Job drawing, mm, ordinate dimensions from the low corner. One solid piece. A direction names the side the tool comes from. Coordinates: 2 decimals unless noted, no trailing zeros. Loops run counter-clockwise (first coordinate to the right, second up) from the corner with the lowest first, then second, coordinate; pieces in that order, holes last. Notation, with made-up numbers: (31, 12) -> (37, 12) arc R32 ccw to (37, 42) -> close; hole circle Ø7 at (68, -21.5). An arc over 180 degrees is marked (long way). Answer as CSV lines item,"result". Start each with the question number.
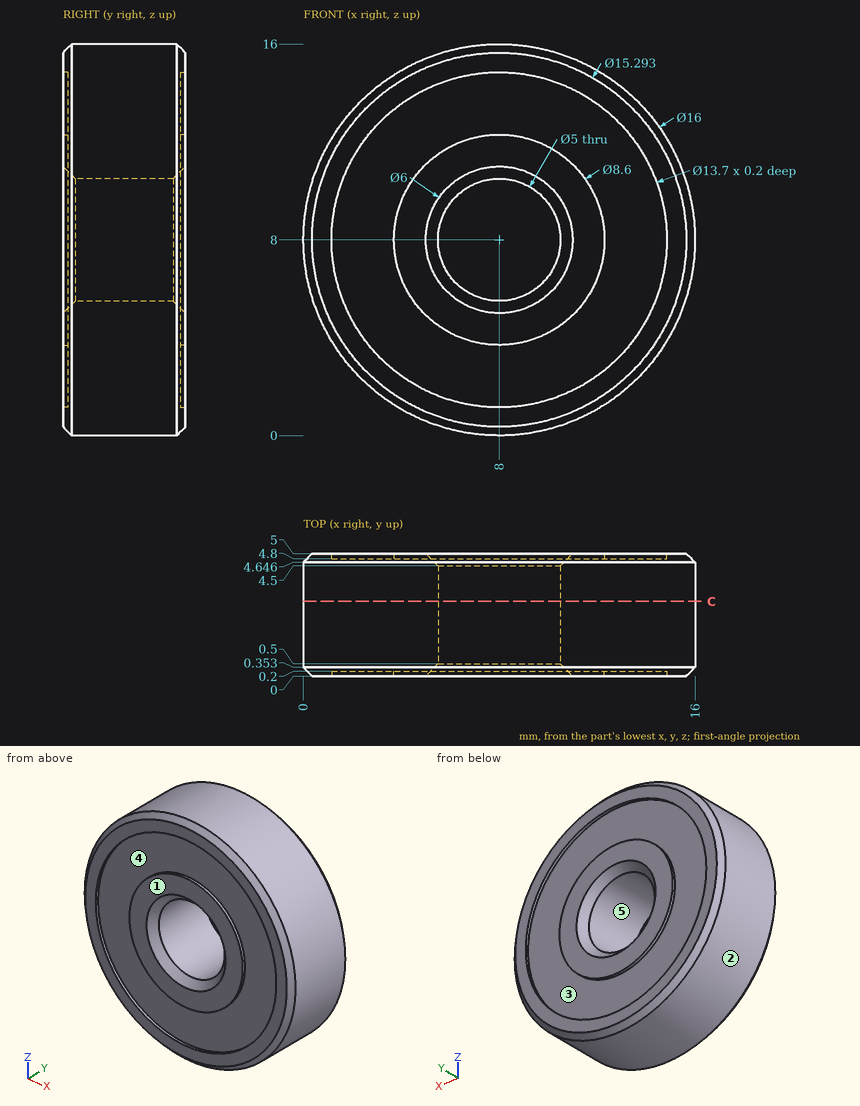
Item 1: Which spindle directions (+Z, -Z, +X, -X, +Y, -Y) get a long thin tool onto all of the face, cutting with end or side? Do the marked faces 4 and 5. Say none if no direction does.
Item 2: Flat gauge pins, fed straight in: pin 1 Ø4 at (x, z) = (8, 8) entering from -Y; pin 2 Ø2 at (x, y) = (5.5, 2.5) entering from -Z; pin 3 Ø3 at (x, y) = (3.5, 3) entering from +Z; pin 4 Ø3 at (y, z) = (2.5, 11.5) entering from -X. Where does each tip first touch, or does it go through?
Item 3: Wall check: probe 1 along Z at (x, y) = (8, 3.3); probe 2 along Y at (x, z) = (13, 12); probe 3 along Z at (x, y) = (10, 2.1) (1 decimal). Give the ranges that are in metal, low to high.
Item 4: Saw through at C-C (y = 3.05). Write the cut outline in (x, z).
Item 5: Two-plate mould, pull along X, no slides. Class the marked faces 1, 2 and 3: pulls with the +X half, pulls with the -X half, needs draft (parallel to the pull), parting line crosses it, or undercut.
Geometry check:
1,face 4,"-Y"
1,face 5,"+Y, -Y"
2,pin 1,"through"
2,pin 2,"z = 0.14"
2,pin 3,"z = 15.42"
2,pin 4,"x = 0.25"
3,probe 1,"0 to 5.5, 10.5 to 16"
3,probe 2,"0.2 to 4.8"
3,probe 3,"0.3 to 6.5, 9.5 to 15.7"
4,outline,"circle Ø16 at (8, 8); hole circle Ø5 at (8, 8)"
5,face 1,"needs draft"
5,face 2,"parting line crosses it"
5,face 3,"undercut"
